Check sheet for the modelled part. Datum: model origin and axes. Units: mm. Coordinates: 2 decimals unless noted, no trailing zeros. Loops run counter-clockwise (first coordinate to the right, second up) from the corner with the lowest first, then second, coordinate; pieces in that order, holes last.
from build123d import *

# Parameters (mm, degrees)
SKETCH1_W                   = 152.4
SKETCH1_H                   = 152.4
SKETCH1_R                   = 17.526
BASE_DEPTH                  = 6.35
F_1_4_0_25_DIAMETER_HOLE1_D = 6.35
CIRPATTERN1_COUNT           = 4


with BuildPart() as part:
    # Sketch1 → Base (new body)
    with BuildSketch(Plane(origin=(0, 0, 0), x_dir=(1, 0, 0), z_dir=(0, 1, 0))):
        Rectangle(SKETCH1_W, SKETCH1_H)
        with Locations(Location((0, 0, 0), (0, 0, 270))):
            Circle(SKETCH1_R, mode=Mode.SUBTRACT)
    extrude(amount=BASE_DEPTH)

    # 1/4 (0.25) Diameter Hole1 (through all)
    with Locations(Plane(origin=(0, 6.35, 0), x_dir=(1, 0, 0), z_dir=(0, 1, 0))):
        with Locations((50.8, -50.8)):
            f_1_4_0_25_diameter_hole1 = Hole(F_1_4_0_25_DIAMETER_HOLE1_D / 2)

    # CirPattern1: 1/4 (0.25) Diameter Hole1 ×4 about axis
    cirpattern1_axis = Axis((0, 0, 0), (0, 1, 0))
    for i in range(1, CIRPATTERN1_COUNT):
        add(f_1_4_0_25_diameter_hole1.rotate(cirpattern1_axis, i * 360 / CIRPATTERN1_COUNT), mode=Mode.SUBTRACT)


solid = part.part
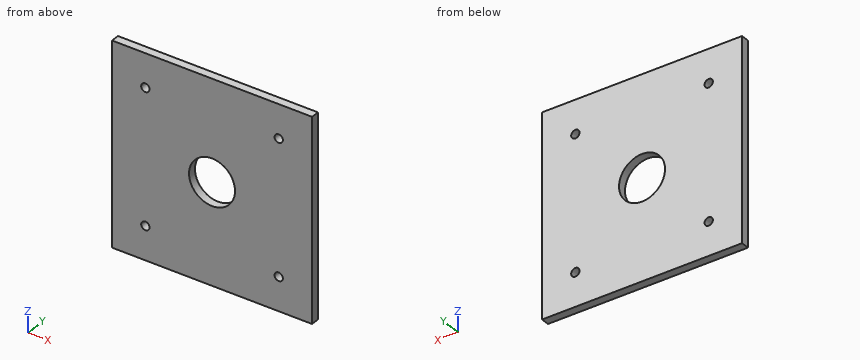
(1) Section check C-C, the plane y = 3. Enter the section's corners in (x, z) (3 decimals), plus the area to 3 significant figures.
(2) Section check D-D, the plane z = 0. Enter the section's corners in (x, y), plus the area to 3 significant figures.
(3) Scan lines: line 1 along Z through (x, y) = (-50.8, 1.5) (3 decimals); line 2 along X through (y, z) = (4.75, -50.5); line 3 along X through (y, z) = (3, 49.5). Record each from-to range of solid material in increasing order.
(4) Section check B-B, the plane z = -50.8. Enter the section's corners in (x, y) (3 decimals).
(5) Gauge pin test, flat end, axial feed: P1, Ø5, axis at x = 50.8, z = -50.8, coming from the +Y side (1 decimal). Record the tip position at first contact, or that the pin passes through.
(6) Section check A-A, the plane x = 0. Enter the section's corners in (y, z).
Determined:
1. outline: (-76.2, -76.2) - (76.2, -76.2) - (76.2, 76.2) - (-76.2, 76.2) - close; hole circle Ø6.35 at (-50.8, -50.8); hole circle Ø6.35 at (-50.8, 50.8); hole circle Ø35.052 at (0, 0); hole circle Ø6.35 at (50.8, -50.8); hole circle Ø6.35 at (50.8, 50.8)
1. area: 22,100 mm2
2. outline: (-76.2, 0) - (-17.53, 0) - (-17.53, 6.35) - (-76.2, 6.35) - close; (17.53, 0) - (76.2, 0) - (76.2, 6.35) - (17.53, 6.35) - close
2. area: 745 mm2
3. line 1: z = -76.2 to -53.975, -47.625 to 47.625, 53.975 to 76.2
3. line 2: x = -76.2 to -53.96, -47.64 to 47.64, 53.96 to 76.2
3. line 3: x = -76.2 to -53.7, -47.9 to 47.9, 53.7 to 76.2
4. outline: (-76.2, 0) - (-53.975, 0) - (-53.975, 6.35) - (-76.2, 6.35) - close; (-47.625, 0) - (47.625, 0) - (47.625, 6.35) - (-47.625, 6.35) - close; (53.975, 0) - (76.2, 0) - (76.2, 6.35) - (53.975, 6.35) - close
5. P1: passes through
6. outline: (0, -76.2) - (6.35, -76.2) - (6.35, -17.53) - (0, -17.53) - close; (0, 17.53) - (6.35, 17.53) - (6.35, 76.2) - (0, 76.2) - close
